The listing builds one solid part. Answer for the finished solid, in the listing's coordinates (mm). A direction names the side the tool comes from. Round coordinates to 2 decimals unless told otherwise and drop trailing zeros. Loops run counter-clockwise (first coordinate to the right, second up) from the corner with the lowest first, then second, coordinate; pieces in that order, holes last. Notation, with made-up numbers: (58, 10.5) -> (71, 10.5) arc R28 ccw to (71, 45.5) -> close; hole circle Ø1 at (18.25, 54.5). An arc over 180 degrees is marked (long way). Answer in a Markdown table with one row per item. Add a question column.
```python
from build123d import *

# Parameters (mm, degrees)
BOSS_EXTRUDE1_DEPTH     = 50
CUT_EXTRUDE1_DEPTH      = 25
SKETCH7_W               = 50
SKETCH7_H               = 50
CUT_EXTRUDE2_DEPTH      = 168.705098312
CUT_EXTRUDE3_DEPTH      = 168.705098312
CUT_EXTRUDE3_DEPTH_BACK = 168.705098312
SKETCH8_R               = 25
CUT_EXTRUDE4_DEPTH      = 168.705098312
CUT_EXTRUDE4_DEPTH_BACK = 168.705098312
SKETCH9_R               = 25
SKETCH15_R              = 25
CUT_EXTRUDE5_DEPTH      = 25


with BuildPart() as part:
    # Sketch2 → Boss-Extrude1 (new, symmetric)
    with BuildSketch(Plane.XY):
        with BuildLine():
            ThreePointArc((-75, 50), (-125, 0), (-75, -50))
            Line((-75, -50), (-75, 50))
        make_face()
        with BuildLine():
            Line((-75, 50), (-75, -50))
            ThreePointArc((-75, -50), (-39.644660941, -35.355339059), (-25, 0))
            ThreePointArc((-25, 0), (-39.644660941, 35.355339059), (-75, 50))
        make_face()
        with BuildLine():
            ThreePointArc((-75, 50), (-125, 0), (-75, -50))
            Line((-75, -50), (-75, 50))
        make_face()
        with BuildLine():
            Line((-75, 50), (-75, -50))
            ThreePointArc((-75, -50), (-39.644660941, -35.355339059), (-25, 0))
            ThreePointArc((-25, 0), (-39.644660941, 35.355339059), (-75, 50))
        make_face()
        with BuildLine():
            ThreePointArc((-25, 0), (-39.644660941, -35.355339059), (-75, -50))
            Line((-75, -50), (75, -50))
            ThreePointArc((75, -50), (25, 0), (75, 50))
            Line((75, 50), (-75, 50))
            ThreePointArc((-75, 50), (-39.644660941, 35.355339059), (-25, 0))
        make_face()
        with BuildLine():
            ThreePointArc((75, 50), (25, 0), (75, -50))
            Line((75, -50), (75, 50))
        make_face()
        with BuildLine():
            Line((75, 50), (75, -50))
            ThreePointArc((75, -50), (110.355339059, -35.355339059), (125, 0))
            ThreePointArc((125, 0), (110.355339059, 35.355339059), (75, 50))
        make_face()
        with BuildLine():
            ThreePointArc((75, 50), (25, 0), (75, -50))
            Line((75, -50), (75, 50))
        make_face()
        with BuildLine():
            Line((75, 50), (75, -50))
            ThreePointArc((75, -50), (110.355339059, -35.355339059), (125, 0))
            ThreePointArc((125, 0), (110.355339059, 35.355339059), (75, 50))
        make_face()
    extrude(amount=BOSS_EXTRUDE1_DEPTH, both=True)

    # Sketch4 → Cut-Extrude1 (cut, symmetric)
    with BuildSketch(Plane.XY):
        with BuildLine():
            Line((-75, -50), (-75, 50))
            ThreePointArc((-75, 50), (-125, 0), (-75, -50))
        make_face()
    extrude(amount=CUT_EXTRUDE1_DEPTH, both=True, mode=Mode.SUBTRACT)

    # Sketch7 → Cut-Extrude2 (cut, through all)
    with BuildSketch(Plane(origin=(0, 50, 0), x_dir=(1, 0, 0), z_dir=(0, 1, 0))):
        with Locations((-50, 0)):
            Rectangle(SKETCH7_W, SKETCH7_H)
    extrude(amount=-CUT_EXTRUDE2_DEPTH, mode=Mode.SUBTRACT)

    # Sketch8 → Cut-Extrude3 (cut, two sides: drawn at the far end of the back side and taken through both)
    with BuildSketch(Plane.XY.offset(50).offset(-CUT_EXTRUDE3_DEPTH_BACK)):
        with Locations((-75, 0)):
            Circle(SKETCH8_R)
    extrude(amount=CUT_EXTRUDE3_DEPTH + CUT_EXTRUDE3_DEPTH_BACK, mode=Mode.SUBTRACT)

    # Sketch9 → Cut-Extrude4 (cut, two sides: drawn at the far end of the back side and taken through both)
    with BuildSketch(Plane.XY.offset(50).offset(-CUT_EXTRUDE4_DEPTH_BACK)):
        with Locations((75, 0)):
            Circle(SKETCH9_R)
    extrude(amount=CUT_EXTRUDE4_DEPTH + CUT_EXTRUDE4_DEPTH_BACK, mode=Mode.SUBTRACT)

    # Sketch15 → Cut-Extrude5 (cut)
    with BuildSketch(Plane.XY.offset(50)):
        with BuildLine():
            Line((75, 50), (25, 50))
            Line((25, 50), (25, -50))
            Line((25, -50), (75, -50))
            ThreePointArc((75, -50), (125, 0), (75, 50))
        make_face()
        with Locations((75, 0)):
            Circle(SKETCH15_R, mode=Mode.SUBTRACT)
    cut_extrude5 = extrude(amount=-CUT_EXTRUDE5_DEPTH, mode=Mode.SUBTRACT)

    # Mirror1: Cut-Extrude5 across plane
    add(cut_extrude5.mirror(Plane.XY), mode=Mode.SUBTRACT)


solid = part.part
```
Item 1: Flat-ended cylindrical pins translate along their axes: P1, Ø5, axis at x = 86, y = 36.5, coming from the +Z side; P2, Ø7.5, axis at y = -10.5, z = 43, coming from the +X side; P3, Ø12, axis at y = 6, z = 11, coming from the +X side. Find the tip coordinate at first contact, or state that the pin passes through.
Item 2: The mould has two halves that part along Z. Classify faces 4 (the cylindrical face through (50.024, 1.099, -0.35)), 5 (the flat face through (-64.6, 22.9, 25)), 6 (the flat face through (-34, 1, -50)), 7 (the flat face through (-25, 1, 0)): +Z half, -Z half, draft (parallel to the pull), parting line (faces both ways), or undercut.
Item 3: For faces 1 (the flat face through (25, 1, 38)), 2 (the flat face through (-64.6, 22.9, -25)), 3 (the flat face through (25, 1, -38)), determine the directions among +Z, -Z, +X, -X, +Y, -Y from which every point of the face is accessible in a straight line to the end or side of a thin tool.
Item 4: Section D-D, the plane y = 40 is taken. Write down the section's boundary in (x, z), and give its area (3 significant figures).
Item 5: Section B-B, the plane x = 56 is taken. Write down the section's boundary in (y, z), and give its area (3 significant figures).
Item 6: Section C-C, the plane z = 34.5 is taken. Write down the section's boundary in (x, y), and give its area (3 significant figures).
Item 7: Section A-A, the plane y = 0 is taken. Write down the section's boundary in (x, z), and give its area (3 significant figures).
Item 8: Consider L1, parallel to Y at x = 75, z = 13; L2, parallel to X at y = -1, z = 30. Determine where each line is inside the solid, lowest interval first. Write a range as from..to.
Here are the results:
| question | item | result |
|---|---|---|
| 1 | P1 | stops at z = 25 |
| 1 | P2 | stops at x = 25 |
| 1 | P3 | stops at x = 125 |
| 2 | face 4 | draft |
| 2 | face 5 | undercut |
| 2 | face 6 | -Z half |
| 2 | face 7 | undercut |
| 3 | face 1 | +Z, +X, +Y, -Y |
| 3 | face 2 | -X, +Y, -Y |
| 3 | face 3 | -Z, +X, +Y, -Y |
| 4 | outline | (-105, -50) -> (25, -50) -> (25, -25) -> (105, -25) -> (105, 25) -> (25, 25) -> (25, 50) -> (-105, 50) -> (-105, 25) -> (-25, 25) -> (-25, -25) -> (-105, -25) -> close |
| 4 | area | 13,000 mm² |
| 5 | outline | (-50, -25) -> (-16.25, -25) -> (-16.25, 25) -> (-50, 25) -> close; (16.25, -25) -> (50, -25) -> (50, 25) -> (16.25, 25) -> close |
| 5 | area | 3,380 mm² |
| 6 | outline | (-75, -50) -> (25, -50) -> (25, 50) -> (-75, 50) arc R50 ccw to start; hole circle Ø50 at (-75, 0) |
| 6 | area | 12,000 mm² |
| 7 | outline | (-125, -50) -> (-100, -50) -> (-100, -25) -> (-125, -25) -> close; (-125, 25) -> (-100, 25) -> (-100, 50) -> (-125, 50) -> close; (-50, -50) -> (25, -50) -> (25, -25) -> (50, -25) -> (50, 25) -> (25, 25) -> (25, 50) -> (-50, 50) -> (-50, 25) -> (-25, 25) -> (-25, -25) -> (-50, -25) -> close; (100, -25) -> (125, -25) -> (125, 25) -> (100, 25) -> close |
| 7 | area | 10,000 mm² |
| 8 | L1 | y = -50..-25, 25..50 |
| 8 | L2 | x = -124.99..-99.98, -50.02..25 |
